Build history of the part. All positions in model axes, mm. A direction names the side the tool comes from. Round coordinates to 2 decimals unless told otherwise and drop trailing zeros. Loops run counter-clockwise (first coordinate to the right, second up) from the corner with the lowest first, then second, coordinate; pieces in that order, holes last. Notation, with made-up numbers: M -23,69 L -19,69 A22 ccw -19,77 Z; hole C 68.25,24.5 d7. An arc over 180 degrees is marked long. One line per item, written item: value.
```python
from build123d import *

# Parameters (mm, degrees)
BOSS_EXTRUDE1_DEPTH = 3
SKETCH2_R           = 2.1
CUT_EXTRUDE1_DEPTH  = 4


with BuildPart() as part:
    # Sketch1 → Boss-Extrude1 (new body)
    with BuildSketch(Plane(origin=(0, 0, 0), x_dir=(1, 0, 0), z_dir=(0, 1, 0))):
        Polygon((15, 0), (20, 0), (20, -50), (23, -50), (23, -100), (20, -100), (20, -150), (0, -150), (0, -100), (-3, -100), (-3, -50), (0, -50), (0, 0), (5, 0), (5, 3), (15, 3), align=None)
    extrude(amount=BOSS_EXTRUDE1_DEPTH)

    # Sketch2 → Cut-Extrude1 (cut, through all)
    with BuildSketch(Plane(origin=(0, 3, 0), x_dir=(1, 0, 0), z_dir=(0, 1, 0))):
        with Locations((10, -7)):
            Circle(SKETCH2_R)
        with Locations((10, -37)):
            Circle(SKETCH2_R)
    extrude(amount=-CUT_EXTRUDE1_DEPTH, mode=Mode.SUBTRACT)


solid = part.part
```
Item 1: Pull direction Z, two halves, no side cores. Call faces 6 (the face through (20, 1, 25)), 7 (the face through (-2, 1, 50)), 8 (the face through (8.452, 1.521, 5.581)), 9 (the face through (8.334, 1.521, 38.278)): pulls with the +Z half, pulls with the -Z half, needs draft (parallel to the pull), parting line crosses it, or undercut.
Check values:
face 6: needs draft
face 7: pulls with the -Z half
face 8: undercut
face 9: undercut
Item 2: Slice it at C-C, the plane y = 1.4. Give the cut face in (x, z).
Check values:
outline: M -3,50 L 0,50 L 0,0 L 5,0 L 5,-3 L 15,-3 L 15,0 L 20,0 L 20,50 L 23,50 L 23,100 L 20,100 L 20,150 L 0,150 L 0,100 L -3,100 Z; hole C 10,7 d4.2; hole C 10,37 d4.2
Item 3: Wall check: line 1 along Z through (x, y) = (10, 2.1); line 2 along X through (y, z) = (2.3, 37); line 3 along X through (y, z) = (2.15, 18.5). Give the ranges that are in metal, low to high.
Check values:
line 1: z = -3 to 4.9, 9.1 to 34.9, 39.1 to 150
line 2: x = 0 to 7.9, 12.1 to 20
line 3: x = 0 to 20
Item 4: Slice it at B-B, the plane x = 10. Give the cut face in (y, z).
Check values:
outline: M 0,-3 L 3,-3 L 3,4.9 L 0,4.9 Z; M 0,9.1 L 3,9.1 L 3,34.9 L 0,34.9 Z; M 0,39.1 L 3,39.1 L 3,150 L 0,150 Z
Item 5: Slice it at D-D, the plane x = 17.5. Give the cut face in (y, z).
Check values:
outline: M 0,0 L 3,0 L 3,150 L 0,150 Z
Item 6: Slice it at A-A, the plane z = 7. Give the cut face in (x, y).
Check values:
outline: M 0,0 L 7.9,0 L 7.9,3 L 0,3 Z; M 12.1,0 L 20,0 L 20,3 L 12.1,3 Z
Item 7: Which spindle directions (+Z, -Z, +X, -X, +Y, -Y) get a long thin tool onto all of the face, cutting with end or side? Do faces 1 (the face through (10, 1, -3)), 2 (the face through (22, 1, 100)), 3 (the face through (-1, 1, 100)), 4 (the face through (5, 1, -1)), 5 (the face through (15, 1, -2)). Say none if no direction does.
Check values:
face 1: -Z, +X, -X, +Y, -Y
face 2: +Z, +X, +Y, -Y
face 3: +Z, -X, +Y, -Y
face 4: -Z, -X, +Y, -Y
face 5: -Z, +X, +Y, -Y
Item 8: Drop flat-ended pins along their axis: P1, Ø0.9, axis at x = 21.5, y = 2, coming from the +Z side; P2, Ø0.9, axis at x = 3, y = 2, coming from the -Z side; P3, Ø0.9, axis at y = 1.5, z = 113.5, coming from the -X side. Give the stop position or say it passes through.
Check values:
P1: stops at z = 100
P2: stops at z = 0
P3: stops at x = 0
